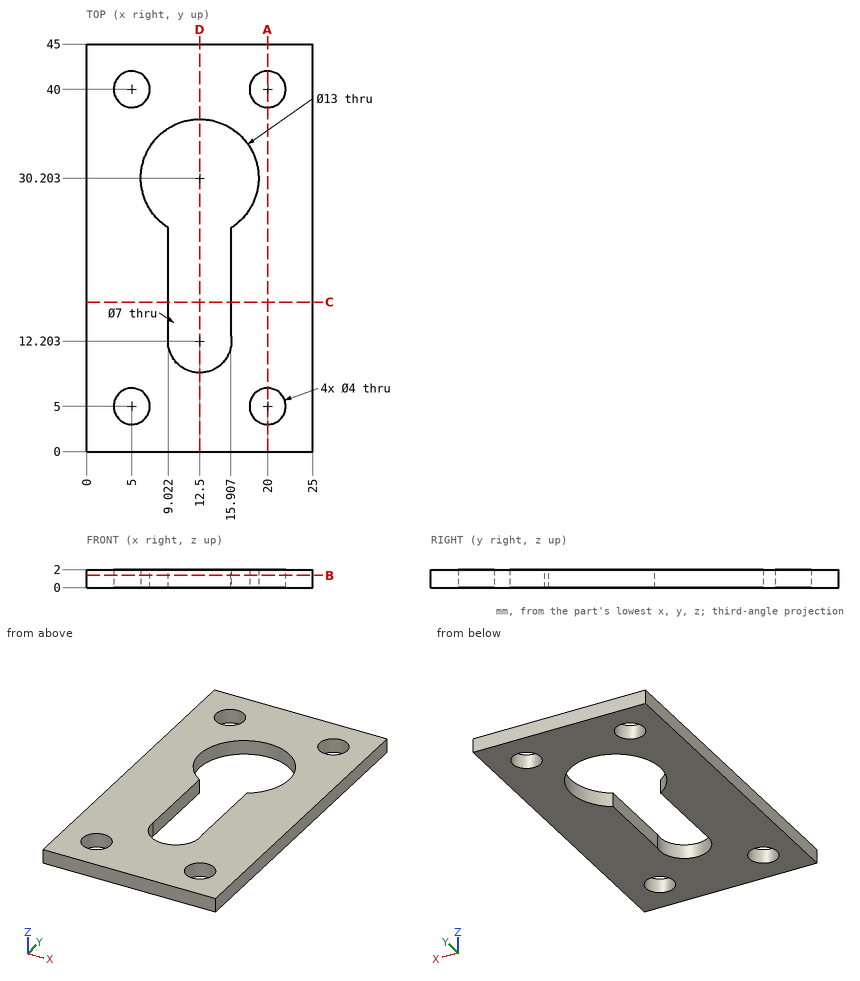
Part print with two shaded views. Sizes in mm from the minimum x, y, z corner. Round coordinates to 2 decimals unless told otherwise and drop trailing zeros. Write each loop counter-clockwise with the first axis right and the second up, starting at its lowest first coordinate (ties: lowest second). Pieces come first, ordered by that corner, then holes. Notation, with made-up numbers: (69.25, 56) -> (76.25, 56) arc R31 cw to (76.25, 92) -> close; hole circle Ø4 at (46.5, 44.25). An arc over 180 degrees is marked (long way). Use one line per item in the form item = value.
Q1. Band-saw the part on A-A, the plane x = 20. Write the cut outline in (y, z).
Conclusion:
outline = (0, 0) -> (3, 0) -> (3, 2) -> (0, 2) -> close; (7, 0) -> (38, 0) -> (38, 2) -> (7, 2) -> close; (42, 0) -> (45, 0) -> (45, 2) -> (42, 2) -> close
Q2. Band-saw the part on D-D, the plane x = 12.5. Write the cut outline in (y, z).
Conclusion:
outline = (0, 0) -> (8.7, 0) -> (8.7, 2) -> (0, 2) -> close; (36.7, 0) -> (45, 0) -> (45, 2) -> (36.7, 2) -> close
Q3. Band-saw the part on C-C, the plane y = 16.5. Write the cut outline in (x, z).
Conclusion:
outline = (0, 0) -> (9.02, 0) -> (9.02, 2) -> (0, 2) -> close; (15.91, 0) -> (25, 0) -> (25, 2) -> (15.91, 2) -> close
Q4. Band-saw the part on B-B, the plane z = 1.35. Write the cut outline in (x, y).
Conclusion:
outline = (0, 0) -> (25, 0) -> (25, 45) -> (0, 45) -> close; hole circle Ø4 at (5, 5); hole circle Ø4 at (5, 40); hole (9.02, 12.59) arc R3.5 ccw (long way) to (15.91, 13) -> (15.91, 24.67) arc R6.5 ccw (long way) to (9.02, 24.71) -> close; hole circle Ø4 at (20, 5); hole circle Ø4 at (20, 40)
Q5. Drill centre lines: L1, parallel to Y at x = 5, z = 0.4; L2, parallel to X at y = 15, z = 0.7; L3, parallel to Y at x = 19.25, z = 1.55 (1 decimal). Where is each one in solid material? Low to high.
Conclusion:
L1 = 0 to 3, 7 to 38, 42 to 45
L2 = 0 to 9.02, 15.91 to 25
L3 = 0 to 3.1, 6.9 to 38.1, 41.9 to 45
